Check sheet for the modelled part. Datum: model origin and axes. Units: mm. A direction names the side the tool comes from. Round coordinates to 2 decimals unless told otherwise and drop trailing zeros. Write each loop counter-clockwise with the first axis right and the second up, starting at its lowest first coordinate (ties: lowest second). Pieces come first, ordered by that corner, then holes. Notation, with made-up numbers: (44.5, 30.25) -> (59.5, 30.25) arc R22 ccw to (59.5, 48.25) -> close; hole circle Ø8 at (69, 11.25). An arc over 180 degrees is marked (long way). One line per item, written item: value. Start each with the question number.
```python
from build123d import *

# Parameters (mm, degrees)
BOSS_EXTRUDE1_DEPTH     = 2.54
BOSS_EXTRUDE2_START     = 54.61
SKETCH2_W               = 28.194
SKETCH2_H               = 28.194
BOSS_EXTRUDE2_DEPTH     = 54.61
SKETCH4_R               = 5.08
CUT_EXTRUDE2_DEPTH      = 1.524
SKETCH5_R               = 2.54
CUT_EXTRUDE3_DEPTH      = 1.016
BOSS_EXTRUDE3_DEPTH     = 17.145
CUT_EXTRUDE4_START      = -7.10691
SKETCH7_R               = 2.794
CUT_EXTRUDE4_DEPTH      = 7.10691
BOSS_EXTRUDE4_DEPTH     = 2.54
BOSS_EXTRUDE5_DEPTH     = 10.16
BOSS_EXTRUDE6_DEPTH     = 19.05
CUT_EXTRUDE5_DEPTH      = 13.716
CUT_EXTRUDE5_DEPTH_BACK = 20.32
SKETCH13_R              = 2.76606
BOSS_EXTRUDE12_DEPTH    = 2.54
SKETCH15_W              = 2.689899245
SKETCH15_H              = 26.801981191
BOSS_EXTRUDE13_DEPTH    = 7.62
BOSS_EXTRUDE14_DEPTH    = 21.082
SKETCH17_R              = 2.54
CUT_EXTRUDE7_DEPTH      = 21.082
CUT_EXTRUDE8_DEPTH      = 21.082


with BuildPart() as part:
    # Sketch1 → Boss-Extrude1 (new body)
    with BuildSketch(Plane(origin=(0, 0, 0), x_dir=(1, 0, 0), z_dir=(0, 1, 0))):
        with BuildLine():
            Line((-11.303, -16.637), (11.303, -16.637))
            ThreePointArc((11.303, -16.637), (15.074707571, -15.074707571), (16.637, -11.303))
            Line((16.637, -11.303), (16.637, 11.303))
            ThreePointArc((16.637, 11.303), (15.074707571, 15.074707571), (11.303, 16.637))
            Line((11.303, 16.637), (-11.303, 16.637))
            ThreePointArc((-11.303, 16.637), (-15.074707571, 15.074707571), (-16.637, 11.303))
            Line((-16.637, 11.303), (-16.637, -11.303))
            ThreePointArc((-16.637, -11.303), (-15.074707571, -15.074707571), (-11.303, -16.637))
        make_face()
    extrude(amount=BOSS_EXTRUDE1_DEPTH)

    # Sketch2 → Boss-Extrude2 (add)
    with BuildSketch(Plane.XZ.offset(BOSS_EXTRUDE2_START)):
        with BuildLine():
            Line((-11.303, 16.637), (11.303, 16.637))
            ThreePointArc((11.303, 16.637), (15.074707571, 15.074707571), (16.637, 11.303))
            Line((16.637, 11.303), (16.637, -11.303))
            ThreePointArc((16.637, -11.303), (15.074707571, -15.074707571), (11.303, -16.637))
            Line((11.303, -16.637), (-11.303, -16.637))
            ThreePointArc((-11.303, -16.637), (-15.074707571, -15.074707571), (-16.637, -11.303))
            Line((-16.637, -11.303), (-16.637, 11.303))
            ThreePointArc((-16.637, 11.303), (-15.074707571, 15.074707571), (-11.303, 16.637))
        make_face()
        Rectangle(SKETCH2_W, SKETCH2_H, mode=Mode.SUBTRACT)
    extrude(amount=-BOSS_EXTRUDE2_DEPTH)

    # Sketch4 → Cut-Extrude2 (cut)
    with BuildSketch(Plane(origin=(0, 0, -16.637), x_dir=(-1, 0, 0), z_dir=(0, 0, -1))):
        with Locations((0, -24.13)):
            Circle(SKETCH4_R)
    extrude(amount=-CUT_EXTRUDE2_DEPTH, mode=Mode.SUBTRACT)

    # Sketch5 → Cut-Extrude3 (cut)
    with BuildSketch(Plane(origin=(0, 0, -15.113), x_dir=(-1, 0, 0), z_dir=(0, 0, -1))):
        with Locations((0, -24.13)):
            Circle(SKETCH5_R)
    extrude(amount=-CUT_EXTRUDE3_DEPTH, mode=Mode.SUBTRACT)

    # Sketch6 → Boss-Extrude3 (add)
    with BuildSketch(Plane(origin=(0, 2.54, 0), x_dir=(1, 0, 0), z_dir=(0, 1, 0))):
        Polygon((5.334, -16.637), (23.168788656, -34.471788656), (28.194132537, -29.446444776), (14.396212982, -15.648525221), align=None)
    extrude(amount=-BOSS_EXTRUDE3_DEPTH)

    # Sketch7 → Cut-Extrude4 (cut)
    with BuildSketch(Plane(origin=(-0.62615612, 0, 0.62615612), x_dir=(-0.7071067811865477, 0, -0.7071067811865475), z_dir=(0.7071067811865475, 0, -0.7071067811865477)).offset(CUT_EXTRUDE4_START)):
        with Locations((-32.249043089, -6.0325)):
            Circle(SKETCH7_R)
    extrude(amount=CUT_EXTRUDE4_DEPTH, mode=Mode.SUBTRACT)

    # Sketch9 → Boss-Extrude4 (add)
    with BuildSketch(Plane(origin=(0, -11.938, 0), x_dir=(1, 0, 0), z_dir=(0, 1, 0))):
        with BuildLine():
            Line((46.562129264, -1.143), (13.310139602, 16.273079187))
            Line((13.310139602, 16.273079187), (12.964036607, 15.721651043))
            Line((12.964036607, 15.721651043), (15.475295461, 12.118791083))
            Line((15.475295461, 12.118791083), (15.475295461, 3.129239018))
            Line((15.475295461, 3.129239018), (15.475295461, 1.47632638))
            ThreePointArc((15.475295461, 1.47632638), (17.263507322, -2.715683033), (21.480153786, -4.445))
            Line((21.480153786, -4.445), (38.24328617, -4.445))
            Line((38.24328617, -4.445), (46.562129264, -4.445))
            Line((46.562129264, -4.445), (46.562129264, -1.143))
        make_face()
    extrude(amount=-BOSS_EXTRUDE4_DEPTH)

    # Sketch10 → Boss-Extrude5 (add)
    with BuildSketch(Plane.XZ.offset(14.478)):
        with BuildLine():
            Line((46.562129264, 1.143), (46.562129264, 4.445))
            Line((46.562129264, 4.445), (21.480153786, 4.445))
            ThreePointArc((21.480153786, 4.445), (18.765347806, 3.796345215), (16.637, 1.990504648))
            Line((16.637, 1.990504648), (16.637, -2.114151714))
            ThreePointArc((16.637, -2.114151714), (18.849336789, 0.264449502), (21.976688198, 1.143))
            Line((21.976688198, 1.143), (46.562129264, 1.143))
        make_face()
    extrude(amount=BOSS_EXTRUDE5_DEPTH)

    # Sketch11 → Boss-Extrude6 (add)
    with BuildSketch(Plane.XZ.offset(24.638)):
        with BuildLine():
            Line((21.976688198, 1.143), (46.562129264, 1.143))
            Line((46.562129264, 1.143), (46.562129264, 4.445))
            Line((46.562129264, 4.445), (46.562129264, 13.843))
            Line((46.562129264, 13.843), (26.43228617, 13.843))
            Line((26.43228617, 13.843), (10.498277863, 16.887218473))
            Line((10.498277863, 16.887218473), (10.837249294, 13.520457424))
            Line((10.837249294, 13.520457424), (26.43228617, 10.541))
            Line((26.43228617, 10.541), (43.387129264, 10.541))
            Line((43.387129264, 10.541), (43.387129264, 4.445))
            Line((43.387129264, 4.445), (21.480153786, 4.445))
            ThreePointArc((21.480153786, 4.445), (18.765347806, 3.796345215), (16.637, 1.990504648))
            Line((16.637, 1.990504648), (16.637, -2.114151714))
            ThreePointArc((16.637, -2.114151714), (18.849336789, 0.264449502), (21.976688198, 1.143))
        make_face()
    extrude(amount=BOSS_EXTRUDE6_DEPTH)

    # Sketch13 → Cut-Extrude5 (cut, two sides: drawn at the far end of the back side and taken through both)
    with BuildSketch(Plane.XY.offset(13.843).offset(-CUT_EXTRUDE5_DEPTH_BACK)):
        with Locations(Location((37.189529264, -34.163, 0), (0, 0, 180))):
            Circle(SKETCH13_R)
    extrude(amount=CUT_EXTRUDE5_DEPTH + CUT_EXTRUDE5_DEPTH_BACK, mode=Mode.SUBTRACT)

    # Sketch14 → Boss-Extrude12 (add)
    with BuildSketch(Plane.XZ.offset(14.605)):
        Polygon((3.404930005, 43.438981191), (0.71503076, 43.438981191), (0.71503076, 16.637), (5.334, 16.637), (11.303, 16.637), (21.779567071, 23.03187931), align=None)
    extrude(amount=-BOSS_EXTRUDE12_DEPTH)

    # Sketch15 → Boss-Extrude13 (add)
    with BuildSketch(Plane.XZ.offset(14.605)):
        with Locations((2.059980383, 30.037990596)):
            Rectangle(SKETCH15_W, SKETCH15_H)
    extrude(amount=BOSS_EXTRUDE13_DEPTH)

    # Sketch16 → Boss-Extrude14 (add)
    with BuildSketch(Plane.XZ.offset(22.225)):
        Polygon((3.404930005, 16.637), (3.404930005, 43.438981191), (-8.406765612, 43.438981191), (-8.406765612, 24.889361191), (-15.692885389, 14.332927767), (-12.390885389, 14.332927767), (-5.104765612, 24.889361191), (-5.104765612, 40.136981191), (0.71503076, 40.136981191), (0.71503076, 16.637), align=None)
    extrude(amount=BOSS_EXTRUDE14_DEPTH)

    # Sketch17 → Cut-Extrude7 (cut)
    with BuildSketch(Plane.ZY.offset(8.406765612)):
        with Locations((34.548981191, -34.417)):
            Circle(SKETCH17_R)
    extrude(amount=-CUT_EXTRUDE7_DEPTH, mode=Mode.SUBTRACT)

    # Sketch18 → Cut-Extrude8 (cut)
    with BuildSketch(Plane.XZ.offset(43.688)):
        Polygon((14.097, 12.897676695), (10.837249294, 13.520457424), (10.779201972, 14.097), (14.097, 14.097), align=None)
    extrude(amount=-CUT_EXTRUDE8_DEPTH, mode=Mode.SUBTRACT)


solid = part.part
```
1. Access from +Z, -Z, +X, -X, +Y, -Y to the whole of each face (thin tool, end or side, straight path). Record for faces 4 (the face through (0.6, -26.6, -14.6)), 5 (the face through (21.404, -34.03, 11.502)), 6 (the face through (30, -11.938, -1)), 7 (the face through (15.12, -26.44, -15.03)).
2. Cross-section at C-C (x = 39). Record the cut outline in (y, z) (3 decimals).
3. Material ranges on probe 1 along Z at (x, y) = (-4, -28); probe 2 along X at (y, z) = (-40.5, -7); probe 3 along Z at (x, y) = (-10.5, -37), recorded low to high.
4. Cross-section at B-B (x = -9.5). Record the cut outline in (y, z) (3 decimals).
5. Cross-section at A-A (z = 9.5). Record the cut outline in (x, y), plus the area to 3 significant figures.
6. Release check for a two-part mould opening along Y. For faces 1 (the face through (-6.78, -36.67, 35.72)), 2 (the face through (18.81, -28.88, 0.24)), 3 (the face through (26, -14.478, -4)) record: +Y half, -Y half, draft (parallel to the pull), parting line (faces both ways), or undercut.
7. Depth check by flat-ended pin: pin 1 Ø3 at (x, y) = (-1.5, -22) entering from -Z; pin 2 Ø7.5 at (x, y) = (30, -29.5) entering from -Z; pin 3 Ø3 at (x, y) = (-5.5, -13.5) entering from +Z. Enter the tip coordinate at first touch or a pass-through.
Working result:
1. face 4: -Z
1. face 5: +Y, -Y
1. face 6: -Z, +X, +Y
1. face 7: -Z, +X
2. outline: (-43.688, 1.143) -> (-36.254, 1.143) -> (-36.254, 4.445) -> (-43.688, 4.445) -> close; (-43.688, 10.541) -> (-36.254, 10.541) -> (-36.254, 13.843) -> (-43.688, 13.843) -> close; (-32.072, 1.143) -> (-14.478, 1.143) -> (-14.478, -2.818) -> (-11.938, -2.818) -> (-11.938, 4.445) -> (-32.072, 4.445) -> close; (-32.072, 10.541) -> (-24.638, 10.541) -> (-24.638, 13.843) -> (-32.072, 13.843) -> close
3. probe 1: z = -16.64 to -14.1, 14.1 to 16.64, 40.14 to 43.44
3. probe 2: x = -16.64 to -14.1, 14.1 to 16.64
3. probe 3: z = -16.64 to -14.1, 14.1 to 16.64, 17.07 to 21.86
4. outline: (-54.61, -16.637) -> (2.54, -16.637) -> (2.54, 16.637) -> (-54.61, 16.637) -> (-54.61, 14.097) -> (0, 14.097) -> (0, -14.097) -> (-54.61, -14.097) -> close; (-43.307, 18.521) -> (-22.225, 18.521) -> (-22.225, 23.305) -> (-43.307, 23.305) -> close
5. outline: (-16.64, -54.61) -> (-14.1, -54.61) -> (-14.1, 0) -> (14.1, 0) -> (14.1, -54.61) -> (16.64, -54.61) -> (16.64, 2.54) -> (-16.64, 2.54) -> close; (43.39, -43.69) -> (46.56, -43.69) -> (46.56, -24.64) -> (43.39, -24.64) -> close
5. area: 422 mm^2
6. face 1: undercut
6. face 2: draft
6. face 3: -Y half
7. pin 1: stops at z = -15.11
7. pin 2: stops at z = 1.14
7. pin 3: stops at z = 16.64
